from build123d import *

# Parameters (mm, degrees)
SKETCH2_W            = 17.272
SKETCH2_H            = 66.675
BOSS_EXTRUDE1_DEPTH  = 12.7
SKETCH3_W            = 5.08
SKETCH3_H            = 6.35
SKETCH3_H_2          = 1.905
SKETCH3_H_3          = 1.27
BOSS_EXTRUDE2_DEPTH  = 12.7
CUT_EXTRUDE1_DEPTH   = 10.16
FILLET2_R            = 3.048
FILLET2_OF_MIRROR1_R = 3.048
CUT_EXTRUDE4_DEPTH   = 70.454139178
CUT_EXTRUDE5_DEPTH   = 0.508
CUT_EXTRUDE6_DEPTH   = 70.454139314


with BuildPart() as part:
    # Sketch2 → Boss-Extrude1 (new body)
    with BuildSketch(Plane(origin=(0, 0, 0), x_dir=(1, 0, 0), z_dir=(0, 1, 0))):
        with Locations((8.636, 33.3375)):
            Rectangle(SKETCH2_W, SKETCH2_H)
    extrude(amount=BOSS_EXTRUDE1_DEPTH)

    # Sketch3 → Boss-Extrude2 (add)
    with BuildSketch(Plane.XZ):
        with Locations((5.08, -29.21)):
            Rectangle(SKETCH3_W, SKETCH3_H)
        with Locations((5.08, -20.955)):
            Rectangle(SKETCH3_W, SKETCH3_H)
        with Locations((5.08, -25.0825)):
            Rectangle(SKETCH3_W, SKETCH3_H_2)
        with Locations((5.08, -33.3375)):
            Rectangle(SKETCH3_W, SKETCH3_H_2)
        with Locations((5.08, -37.465)):
            Rectangle(SKETCH3_W, SKETCH3_H)
        with Locations((5.08, -41.275)):
            Rectangle(SKETCH3_W, SKETCH3_H_3)
    extrude(amount=BOSS_EXTRUDE2_DEPTH)

    # Sketch4 → Cut-Extrude1 (cut)
    with BuildSketch(Plane.XY):
        Polygon((0, 7.62), (5.3975, 7.62), (5.3975, 12.7), (11.8745, 12.7), (11.8745, 7.62), (17.272, 7.62), (17.272, 2.794), (0, 2.794), align=None)
    cut_extrude1 = extrude(amount=-CUT_EXTRUDE1_DEPTH, mode=Mode.SUBTRACT)

    # Fillet2
    fillet2_edges = [part.edges().sort_by_distance(p)[0] for p in [
        (5.3975, 10.16, -10.16),
        (11.8745, 10.16, -10.16),
    ]]
    fillet(fillet2_edges, radius=FILLET2_R)

    # Mirror1: Cut-Extrude1 across plane
    add(cut_extrude1.mirror(Plane.XY.offset(-33.3375)), mode=Mode.SUBTRACT)

    # Fillet2 of Mirror1
    fillet2_of_mirror1_edges = [part.edges().sort_by_distance(p)[0] for p in [
        (5.3975, 10.16, -56.515),
        (11.8745, 10.16, -56.515),
    ]]
    fillet(fillet2_of_mirror1_edges, radius=FILLET2_OF_MIRROR1_R)

    # Sketch5 → Cut-Extrude4 (cut, through all)
    with BuildSketch(Plane.ZY.offset(-2.54)):
        with BuildLine():
            Line((-66.675, -12.7), (0, -12.7))
            ThreePointArc((0, -12.7), (-33.3375, -10.668), (-66.675, -12.7))
        make_face()
    extrude(amount=-CUT_EXTRUDE4_DEPTH, mode=Mode.SUBTRACT)

    # Sketch6 → Cut-Extrude5 (cut)
    with BuildSketch(Plane(origin=(0, 12.7, 0), x_dir=(1, 0, 0), z_dir=(0, 1, 0))):
        with BuildLine():
            Line((5.776894531, 32.530175781), (6.185, 32.690136719))
            Line((6.185, 32.690136719), (6.185, 34.051171875))
            Line((6.185, 34.051171875), (5.768007812, 34.211132812))
            add(Edge.make_bspline(
                [(5.768007812, 34.211132812), (5.730494518, 34.225820978), (5.661738716, 34.25274201), (5.569524922, 34.294468396), (5.496856289, 34.332290336), (5.44041907, 34.367362499), (5.398808713, 34.408271263), (5.372150366, 34.459568119), (5.356449781, 34.520790431), (5.354690345, 34.564901212), (5.35375, 34.588476562)],
                knots=[0, 0, 0, 0, 1.589179946, 2.912709847, 3.990397165, 4.820646782, 5.526248733, 6.26234321, 7.071295771, 8, 8, 8, 8], degree=3))
            add(Edge.make_bspline(
                [(5.35375, 34.588476562), (5.354923711, 34.609350692), (5.35723832, 34.650515396), (5.376105038, 34.709983847), (5.405904793, 34.765474392), (5.446909477, 34.815335315), (5.494806824, 34.85769508), (5.547709989, 34.88945387), (5.604426015, 34.909062179), (5.643671152, 34.911349233), (5.663417969, 34.9125)],
                knots=[0, 0, 0, 0, 1.012851797, 1.997388367, 3.003373292, 4.058581268, 5.118255936, 6.09654221, 7.042244815, 8, 8, 8, 8], degree=3))
            add(Edge.make_bspline(
                [(5.663417969, 34.9125), (5.687013914, 34.911555345), (5.735537805, 34.90961271), (5.796155547, 34.892709958), (5.849374825, 34.875661052), (5.897051464, 34.858225338), (5.952411749, 34.838064341), (5.991361751, 34.822388839), (6.012050781, 34.8140625)],
                knots=[0, 0, 0, 0, 1.162954171, 2.391557502, 3.08930458, 3.926034863, 4.898374222, 6, 6, 6, 6], degree=3))
            Line((6.012050781, 34.8140625), (8.209804687, 33.957519531))
            add(Edge.make_bspline(
                [(8.209804687, 33.957519531), (8.226428771, 33.951113113), (8.261020453, 33.937782526), (8.315677882, 33.917334175), (8.374470369, 33.893962658), (8.436973219, 33.870121703), (8.499246191, 33.845277035), (8.557274142, 33.8177815), (8.609899907, 33.789999082), (8.657389954, 33.761144082), (8.699684296, 33.729310109), (8.738099697, 33.693741829), (8.770436623, 33.651946673), (8.800403384, 33.607060747), (8.824677671, 33.556645473), (8.841672776, 33.500421669), (8.85196969, 33.4385942), (8.85314235, 33.395419307), (8.85375, 33.373046875)],
                knots=[0, 0, 0, 0, 0.906379869, 1.886010981, 2.968854674, 4.124928175, 5.289572165, 6.378603586, 7.389892814, 8.31643566, 9.202117826, 10.079567999, 10.970318812, 11.883493671, 12.821997982, 13.804710887, 14.862441745, 16, 16, 16, 16], degree=3))
            add(Edge.make_bspline(
                [(8.85375, 33.373046875), (8.853143023, 33.350446171), (8.85197131, 33.306817548), (8.841657146, 33.244325061), (8.824718356, 33.187386785), (8.800407201, 33.136711098), (8.771490665, 33.091190553), (8.738270432, 33.050541152), (8.70140971, 33.013950972), (8.646096874, 32.972422303), (8.570937447, 32.928580779), (8.490808779, 32.890179852), (8.419869551, 32.862917705), (8.358755001, 32.838536673), (8.289151734, 32.812137701), (8.23988638, 32.793577043), (8.21390625, 32.783789062)],
                knots=[0, 0, 0, 0, 1.00520059, 1.940449142, 2.809766755, 3.639873923, 4.433178694, 5.204465738, 5.971742598, 6.738416121, 8.27578173, 9.83615209, 10.687299641, 11.65709467, 12.764466697, 14, 14, 14, 14], degree=3))
            Line((8.21390625, 32.783789062), (6.030507812, 31.908789062))
            add(Edge.make_bspline(
                [(6.030507812, 31.908789062), (6.010470664, 31.900780275), (5.971885996, 31.885358101), (5.916134993, 31.863706725), (5.864078369, 31.847042494), (5.816554299, 31.832321275), (5.773278478, 31.820653382), (5.734277438, 31.812380787), (5.699571652, 31.807024394), (5.67778988, 31.806498136), (5.667519531, 31.80625)],
                knots=[0, 0, 0, 0, 1.366342978, 2.631107437, 3.785388659, 4.825962469, 5.781334485, 6.621722106, 7.350126631, 8, 8, 8, 8], degree=3))
            add(Edge.make_bspline(
                [(5.667519531, 31.80625), (5.648226041, 31.807426445), (5.609433355, 31.809791878), (5.553209022, 31.829532937), (5.499526082, 31.860395105), (5.450055079, 31.902282304), (5.40703675, 31.952295628), (5.376604178, 32.009857625), (5.357023182, 32.071819825), (5.354854098, 32.115086145), (5.35375, 32.137109375)],
                knots=[0, 0, 0, 0, 0.918866393, 1.847529694, 2.812122199, 3.862154056, 4.927509125, 5.939679135, 6.951264583, 8, 8, 8, 8], degree=3))
            add(Edge.make_bspline(
                [(5.35375, 32.137109375), (5.354800528, 32.162129105), (5.356770672, 32.209050699), (5.378297511, 32.273936), (5.412022157, 32.327652709), (5.44901113, 32.36544648), (5.485613066, 32.391416915), (5.519260812, 32.411831411), (5.559015285, 32.432959548), (5.618650091, 32.460955232), (5.691860724, 32.493644584), (5.749980868, 32.518613458), (5.776894531, 32.530175781)],
                knots=[0, 0, 0, 0, 1.202442774, 2.255041588, 3.251816137, 4.238368336, 4.781120761, 5.412282472, 6.134737701, 6.950402798, 8.587824681, 10, 10, 10, 10], degree=3))
        make_face()
        Polygon((6.71, 33.8734375), (6.71, 32.87265625), (8.11, 33.377832031), align=None, mode=Mode.SUBTRACT)
    extrude(amount=-CUT_EXTRUDE5_DEPTH, mode=Mode.SUBTRACT)

    # Sketch7 → Cut-Extrude6 (cut, through all)
    with BuildSketch(Plane.ZY.offset(-2.54)):
        with BuildLine():
            Line((-17.78, -11.109241116), (-17.78, -10.805360899))
            Line((-17.78, -10.805360899), (-30.099808499, -10.687095595))
            ThreePointArc((-30.099808499, -10.687095595), (-23.93753417, -10.829000448), (-17.78, -11.109241116))
        make_face()
    extrude(amount=-CUT_EXTRUDE6_DEPTH, mode=Mode.SUBTRACT)


solid = part.part
Design review of the part built by this model. Coordinates are the model's own, in mm. A direction names the side the tool comes from. Give positions to 0.01 mm unless a question says otherwise; leave off trailing zeros. Loops run counter-clockwise (first coordinate to the right, second up) from the corner with the lowest first, then second, coordinate; pieces in that order, holes last. Notation, with made-up numbers: M -20,5.5 L 29,5.5 A11 ccw 29,23.5 Z; hole C -27,-5.5 d3. An arc over 180 degrees is marked long. Answer as a JSON object with one key per item and string values.
Item 1: Mouldability with a two-part tool opening along Y and no side actions: class faces 1 (the face through (5.398, 10, -63)), 2 (the face through (9, 2.794, -5)) as pulls with the +Y half, pulls with the -Y half, needs draft (parallel to the pull), parting line crosses it, or undercut.
Output values:
{"face 1": "needs draft", "face 2": "undercut"}
Item 2: We need section A-A (z = -5). State the section outline as (x, y) points.
Output values:
{"outline": "M 0,0 L 17.27,0 L 17.27,2.79 L 0,2.79 Z; M 0,7.62 L 5.4,7.62 L 5.4,12.7 L 0,12.7 Z; M 11.87,7.62 L 17.27,7.62 L 17.27,12.7 L 11.87,12.7 Z"}
Item 3: Wall thickness on line 1 along X through (y, z) = (7.75, -62); line 2 along Y through (x, z) = (8.75, -17); line 3 along Z through (x, y) = (16.5, 3.75) (3 decimals): over which ranges is each line inside the solid? List them lowest first.
Output values:
{"line 1": "x = 0 to 5.4, 11.87 to 17.27", "line 2": "y = 0 to 12.7", "line 3": "z = -56.515 to -10.16"}
Item 4: Machinability: for faces 3 (the face through (10.958, 10.124, -57.384)), 4 (the face through (5.398, 10, -4)), 5 (the face through (7.62, -5, -30)), 6 (the face through (2.54, -5, -30)), which of the approach directions +Z, -Z, +X, -X, +Y, -Y give a long, thin tool a straight path to every point of the face, cutting with its end or side? Answer none if there is none.
Output values:
{"face 3": "-Z, +Y", "face 4": "+Z, +Y", "face 5": "+Z, -Z, +X, -Y", "face 6": "+Z, -Z, -X, -Y"}
Item 5: For P1, Ø4, axis at x = 11.5, z = -59.5, coming from the -Y side; P2, Ø1.5, axis at x = 4.5, z = -34.5, coming from the -Y side; P3, Ø5.5, axis at y = -3.5, z = -32, coming from the -X side, all flat-tipped, find the tip position at first contact; note any pin that passes through.
Output values:
{"P1": "stops at y = 0", "P2": "stops at y = -10.67", "P3": "stops at x = 2.54"}
Item 6: We need section D-D (z = -20.5). State the section outline as (x, y) points.
Output values:
{"outline": "M 0,0 L 2.54,0 L 2.54,-10.78 L 7.62,-10.78 L 7.62,0 L 17.27,0 L 17.27,12.7 L 0,12.7 Z"}
Item 7: We need section C-C (x = 1.5). State the section outline as (y, z) points (3 decimals).
Output values:
{"outline": "M 0,-66.675 L 2.794,-66.675 L 2.794,-56.515 L 7.62,-56.515 L 7.62,-66.675 L 12.7,-66.675 L 12.7,0 L 7.62,0 L 7.62,-10.16 L 2.794,-10.16 L 2.794,0 L 0,0 Z"}
